```python
from build123d import *

# Parameters (mm, degrees)
F1_DEPTH  = 19.05
F2_R      = 6.35
F3_DEPTH  = 19.051
F2_R_2    = 11.176
F4_DEPTH  = 6.35
F5_R      = 25.4
F6_DEPTH  = 31.75
F7_R      = 14.351
F8_DEPTH  = 50.801
F10_W     = 12.7
F10_H     = 19.05
F11_DEPTH = 120.651
F13_W     = 12.7
F13_H     = 19.05
F14_DEPTH = 77.471


with BuildPart() as f1:
    # F0 (on Top) → F1 (new body)
    with BuildSketch(Plane.XY):
        with BuildLine():
            Line((44.45, 25.4), (-44.45, 25.4))
            ThreePointArc((-44.45, 25.4), (-69.85, 0), (-44.45, -25.4))
            Line((-44.45, -25.4), (44.45, -25.4))
            ThreePointArc((44.45, -25.4), (69.85, 0), (44.45, 25.4))
        make_face()
    extrude(amount=-F1_DEPTH)

    # F2 (on face) → F3 (cut, through all)
    with BuildSketch(Plane.XY):
        with Locations((-44.45, 0)):
            Circle(F2_R)
        with Locations((44.45, 0)):
            Circle(F2_R)
    extrude(amount=-F3_DEPTH, mode=Mode.SUBTRACT)

    # F2 (on face) → F4 (cut)
    with BuildSketch(Plane.XY):
        with Locations((-44.45, 0)):
            Circle(F2_R_2)
        with Locations((-44.45, 0)):
            Circle(F2_R, mode=Mode.SUBTRACT)
        with Locations((44.45, 0)):
            Circle(F2_R_2)
        with Locations((44.45, 0)):
            Circle(F2_R, mode=Mode.SUBTRACT)
    extrude(amount=-F4_DEPTH, mode=Mode.SUBTRACT)

    # F5 (on face) → F6 (join)
    with BuildSketch(Plane.XY):
        Circle(F5_R)
    extrude(amount=F6_DEPTH)

    # F7 (on face) → F8 (cut, through all)
    with BuildSketch(Plane.XY.offset(31.75)):
        Circle(F7_R)
    extrude(amount=-F8_DEPTH, mode=Mode.SUBTRACT)

    # F10 (on offset) → F11 (cut, through all)
    with BuildSketch(Plane.YZ.offset(50.8)):
        with Locations((0, 22.225)):
            Rectangle(F10_W, F10_H)
    extrude(amount=-F11_DEPTH, mode=Mode.SUBTRACT)

    # F13 (on offset) → F14 (cut, through all)
    with BuildSketch(Plane.XZ.offset(52.07)):
        with Locations((0, 22.225)):
            Rectangle(F13_W, F13_H)
    extrude(amount=-F14_DEPTH, mode=Mode.SUBTRACT)


solid = f1.part
```
The model under review builds one solid part; all positions refer to its coordinate system, in mm. A direction names the side the tool comes from. Give positions to 0.01 mm unless a question says otherwise; leave off trailing zeros. Write each loop counter-clockwise with the first axis right and the second up, starting at its lowest first coordinate (ties: lowest second). Pieces come first, ordered by that corner, then holes. Notation, with made-up numbers: M 15.5,-27 L 53.5,-27 A32 ccw 53.5,8 Z; hole C 56.5,18.5 d9. An arc over 180 degrees is marked long. Write each question's results on one line, items separated by ' | '. Start each with the question number.
1. Insertion check: pin 1 Ø3.5 at (y, z) = (17, 22) entering from -X; pin 2 Ø9.5 at (x, z) = (-16.5, 21) entering from -Y; pin 3 Ø18 at (x, y) = (43.5, -3) entering from +Z; pin 4 Ø14 at (x, y) = (2.5, 20.5) entering from +Z. Each pin has a flat end and moves straight along its axis. Give the tip position at first contact, or say it passes through.
2. We need section B-B (y = 0). Write out the cut boundary in (x, z), and give its area (3 significant figures).
3. Mouldability with a two-part tool opening along Y and no side actions: class faces 1 (the flat face through (34, 6, 0)), 2 (the cylindrical face through (24.227, 7.629, 15.653)), 3 (the flat face through (-40, -5, -6.35)) as released by +Y, released by -Y, zero draft, split by the parting line, or undercut.
4. We need section C-C (x = 16). Write out the cut boundary in (y, z).
5. For probe 1 along Y at (x, z) = (-44.45, -14.5); probe 2 along Y at (x, z) = (0, -2.5); probe 3 along X at (y, z) = (-4, -7), list the stretches that pass through material, from the lowest coordinate up. Write a range as [from, to].
6. We need section A-A (z = 20.5). Write out the cut boundary in (x, y), and give its area (3 significant figures).
7. We need section D-D (z = 6). Write out the cut boundary in (x, y), and give its area (3 significant figures).
8. For faces 4 (the flat face through (6.35, -19, 22)), 5 (the flat face through (19, 0, 12.7)), 6 (the cylindrical face through (-14.337, 0.631, 1.061)), list the 3-axis set-ups (+Z, -Z, +X, -X, +Y, -Y) from which the entire face can be reached by the end or side of a thin tool; tool diameter is ignored.
Results found:
1) pin 1: stops at x = -20.31 | pin 2: stops at y = -22.52 | pin 3: stops at z = 0 | pin 4: stops at z = 31.75
2) outline: M -69.85,-19.05 L -50.8,-19.05 L -50.8,-6.35 L -55.63,-6.35 L -55.63,0 L -69.85,0 Z; M -38.1,-19.05 L -14.35,-19.05 L -14.35,12.7 L -25.4,12.7 L -25.4,0 L -33.27,0 L -33.27,-6.35 L -38.1,-6.35 Z; M 14.35,-19.05 L 38.1,-19.05 L 38.1,-6.35 L 33.27,-6.35 L 33.27,0 L 25.4,0 L 25.4,12.7 L 14.35,12.7 Z; M 50.8,-19.05 L 69.85,-19.05 L 69.85,0 L 55.63,0 L 55.63,-6.35 L 50.8,-6.35 Z | area: 1,790 mm^2
3) face 1: zero draft | face 2: split by the parting line | face 3: undercut
4) outline: M -25.4,-19.05 L 25.4,-19.05 L 25.4,0 L 19.73,0 L 19.73,31.75 L 6.35,31.75 L 6.35,12.7 L -6.35,12.7 L -6.35,31.75 L -19.73,31.75 L -19.73,0 L -25.4,0 Z
5) probe 1: y = [-25.4, -6.35], [6.35, 25.4] | probe 2: y = [-25.4, -14.35], [14.35, 25.4] | probe 3: x = [-69.53, -49.38], [-39.52, -13.78], [13.78, 39.52], [49.38, 69.53]
6) outline: M -24.59,-6.35 A25.4 ccw -6.35,-24.59 L -6.35,-12.87 A14.35 cw -12.87,-6.35 Z; M -24.59,6.35 L -12.87,6.35 A14.35 cw -6.35,12.87 L -6.35,24.59 A25.4 ccw Z; M 6.35,-24.59 A25.4 ccw 24.59,-6.35 L 12.87,-6.35 A14.35 cw 6.35,-12.87 Z; M 6.35,12.87 A14.35 cw 12.87,6.35 L 24.59,6.35 A25.4 ccw 6.35,24.59 Z | area: 808 mm^2
7) outline: C 0,0 d50.8; hole C 0,0 d28.7 | area: 1,380 mm^2
8) face 4: +Z, +Y, -Y | face 5: +Z, +X, -X | face 6: +Z, -Z
